The listing builds one solid part. Answer for the finished solid, in the listing's coordinates (mm). A direction names the side the tool comes from. Coordinates: 2 decimals unless noted, no trailing zeros. Order: outer loops, then holes, each group sorted by start corner. A loop starts at its lowest first (then second) coordinate and runs counter-clockwise, first axis right, second up. Notation, with made-up numbers: (-23, 87) -> (11, 87) arc R20 ccw to (11, 112) -> close; hole circle Ø8 at (-28, -3). An arc over 180 degrees is marked (long way). Put each result on its own line as item: value. Start each with the question number.
Autodesk Inventor part; units mm, degrees
ref_plane "YZ Plane" through (0, 0, 0) normal (1, 0, 0) x (0, 1, 0)
ref_plane "XZ Plane" through (0, 0, 0) normal (0, 1, 0) x (-1, 0, 0)
ref_plane "XY Plane" through (0, 0, 0) normal (0, 0, 1) x (1, 0, 0)
sketch "Sketch1" plane through (0, 0, 0) normal (0, 0, 1) x (1, 0, 0)
  circle A0 centre (0, 0) radius 29
  dimension "d0" = 58
extrude "Extrusion1" add sketch "Sketch1" along normal blind 3
sketch "Sketch2" plane through (0, 0, 3) normal (0, 0, 1) x (1, 0, 0)
  circle A0 centre (0, 0) radius 2
  dimension "d3" = 4
extrude "Extrusion2" add sketch "Sketch2" along normal blind 24
sketch "Sketch3" plane through (0, 0, 27) normal (0, 0, 1) x (1, 0, 0)
  circle A0 centre (0, 0) radius 29
  dimension "d6" = 58
extrude "Extrusion3" add sketch "Sketch3" along normal blind 1
sketch "Sketch4" plane through (0, 0, 28) normal (0, 0, 1) x (1, 0, 0)
  circle A0 centre (0, 0) radius 1.1
  dimension "d9" = 2.2
extrude "Extrusion4" cut sketch "Sketch4" against normal through all
sketch "Sketch6" plane through (0, 0, 28) normal (0, 0, 1) x (1, 0, 0)
  circle A0 centre (0, 0) radius 2 construction
  circle A1 centre (-16.8114, -22.5) radius 0.4
  circle A2 centre (-2.5, 0) radius 0.4
  circle A3 centre (0, 0) radius 29
  dimension "d20" = 0.8
  dimension "d21" = 0.8
  dimension "d32" = 2.5
  dimension "d41" = 22.5
sketch "Sketch7" plane through (0, 0, 28) normal (0, 0, 1) x (1, 0, 0)
  point P0 (0, 0)
extrude "Extrusion5" cut sketch "Sketch6" against normal up to surface (1 mm away) contours A1 | A2
chamfer "Chamfer1" distance 0.4 angle 45 2 edges at (-2.9, 0, 28) (-17.2114, -22.5, 28)
sketch "Sketch9" plane through (0, 0, 0) normal (0, 0, -1) x (-1, 0, 0)
  point P0 (0, 0)
  point P1 (11, -11.5)
  point P2 (-11, -11.5)
  point P3 (11, -16.5)
  point P4 (-11, -16.5)
  dimension "d44" = 11
  dimension "d45" = 11
  dimension "d46" = 11.5
  dimension "d47" = 11.5
  dimension "d48" = 5
  dimension "d49" = 5
hole "Hole2" at (11, -11.5, 0) at (-11, -11.5, 0) at (-11, -16.5, 0) at (11, -16.5, 0) direction (0, 0, 1) diameter 2.459 depth 2.8
loft "Loft1" [suppressed]
properties part number "Bobbin_x_b"
(1) A tool of negligible diameter and unlimited length cuts with its end or side. For faces 1 (the cylindrical face through (0, 2, 15)), 2 (the flat face through (6, 0, 0)), 3 (the flat face through (11, -17, 2.8)), from which of +Z, -Z, +X, -X, +Y, -Y can it reach the whole face along a straight path? Write none if from no direction.
(2) Each of these flat-tipped pins is pushed along its axis until it touches: P1, Ø10, axis at x = 6.5, z = 19.5, coming from the +Y side; P2, Ø0.7, axis at x = -11, y = -16.5, coming from the -Z side; P3, Ø12, axis at x = -16, z = 11.5, coming from the -Y side; P4, Ø2.5, axis at x = 11, y = -12, coming from the -Z side. Where does it stop, or does it pass through?
(3) The part is cut by section A-A on x = 0. Determine the outline of the cut face in (y, z), plus the area to 3 significant figures.
(4) The part is cut by section C-C on z = 9.25. Determine the outline of the cut face in (x, y).
(5) Find the intervals of material crossed by L1, parallel to Z at x = 20.5, y = 19; L2, parallel to Y at x = -11, z = 0.6; L3, parallel to Y at x = 0, z = 19.5, in increasing order.
(6) The part is cut by section B-B on y = -11.5. Determine the outline of the cut face in (x, z).
(7) The part is cut by section D-D on x = -13. Determine the outline of the cut face in (y, z).
(8) For a pull along Z with two mould halves and no side action, classify faces 4 (the flat face through (6, 0, 3)), 5 (the flat face through (-11, -12, 2.8)), 6 (the cylindrical face through (13.38, 25.73, 1.48)) as released by +Z, released by -Z, zero draft, split by the parting line, or undercut.
Worked out:
1. face 1: none
1. face 2: -Z, +X, -X, +Y, -Y
1. face 3: -Z
2. P1: y = 1.32
2. P2: z = 2.8
2. P3: through
2. P4: z = 0
3. outline: (-29, 0) -> (-1.1, 0) -> (-1.1, 28) -> (-29, 28) -> (-29, 27) -> (-2, 27) -> (-2, 3) -> (-29, 3) -> close; (1.1, 0) -> (29, 0) -> (29, 3) -> (2, 3) -> (2, 27) -> (29, 27) -> (29, 28) -> (1.1, 28) -> close
3. area: 266 mm2
4. outline: circle Ø4 at (0, 0); hole circle Ø2.2 at (0, 0)
5. L1: 0 to 3, 27 to 28
5. L2: -26.83 to -17.73, -15.27 to -12.73, -10.27 to 26.83
5. L3: -2 to -1.1, 1.1 to 2
6. outline: (-26.62, 0) -> (-12.23, 0) -> (-12.23, 2.8) -> (-9.77, 2.8) -> (-9.77, 0) -> (9.77, 0) -> (9.77, 2.8) -> (12.23, 2.8) -> (12.23, 0) -> (26.62, 0) -> (26.62, 3) -> (-26.62, 3) -> close; (-26.62, 27) -> (26.62, 27) -> (26.62, 28) -> (-26.62, 28) -> close
7. outline: (-25.92, 0) -> (25.92, 0) -> (25.92, 3) -> (-25.92, 3) -> close; (-25.92, 27) -> (25.92, 27) -> (25.92, 28) -> (-25.92, 28) -> close
8. face 4: undercut
8. face 5: released by -Z
8. face 6: zero draft
